from build123d import *

# Parameters (mm, degrees)
F1_DEPTH = 2
F3_DEPTH = 35
F5_DEPTH = 2


with BuildPart() as f1:
    # F0 (on Top) → F1 (new body)
    with BuildSketch(Plane.XY):
        Polygon((-94, 0), (94, 0), (0, 89.7997772826), align=None)
    extrude(amount=F1_DEPTH)

    # F2 (on face) → F3 (join)
    with BuildSketch(Plane.XY.offset(2)):
        Polygon((-91.1046698793, 0), (0, 87.0338198358), (91.1046698793, 0), (94, 0), (0, 89.7997772826), (-94, 0), align=None)
    extrude(amount=F3_DEPTH)

    # F4 (on face) → F5 (join)
    with BuildSketch(Plane.XY.offset(37)):
        Polygon((-91.1046698793, 0), (91.1046698793, 0), (0, 87.0338198358), align=None)
        Polygon((91.1046698793, 0), (94, 0), (0, 89.7997772826), (-94, 0), (-91.1046698793, 0), (0, 87.0338198358), align=None)
    extrude(amount=F5_DEPTH)


solid = f1.part
Build history of the part. All positions in model axes, mm. A direction names the side the tool comes from. Give positions to 0.01 mm unless a question says otherwise; leave off trailing zeros. Order: outer loops, then holes, each group sorted by start corner. A loop starts at its lowest first (then second) coordinate and runs counter-clockwise, first axis right, second up. Notation, with made-up numbers: M 62,-39.5 L 115,-39.5 A14 ccw 115,-35.5 Z; hole C -8.75,-18.75 d5. An arc over 180 degrees is marked long. Put each result on its own line as item: value.
Item 1: Drop flat-ended pins along their axis: pin 1 Ø8 at (y, z) = (10.5, 31.5) entering from -X; pin 2 Ø1 at (y, z) = (73.5, 26) entering from +X; pin 3 Ø6 at (y, z) = (74, 18) entering from -X. Give the stop position or say it passes through.
Results are:
pin 1: x = -87.2
pin 2: x = 17.59
pin 3: x = -19.68
Item 2: Cut at B-B on z = 9. Write the cut outline in (x, y).
Results are:
outline: M -94,0 L -91.1,0 L 0,87.03 L 91.1,0 L 94,0 L 0,89.8 Z
Item 3: Cut at D-D on y = 25. Write the cut outline in (x, z), then the cut area to 3 significant figures.
Results are:
outline: M -67.83,0 L 67.83,0 L 67.83,39 L -67.83,39 Z; hole M -64.94,2 L 64.94,2 L 64.94,37 L -64.94,37 Z
area: 745 mm2
Item 4: Which spindle directions (+Z, -Z, +X, -X, +Y, -Y) get a long thin tool onto all of the face, cutting with end or side? Do faces 5 (the face through (-46.2, 42.9, 19.3)), 6 (the face through (-1, 36, 0)). Say none if no direction does.
Results are:
face 5: -Y
face 6: -Z, +X, -X, +Y, -Y
Item 5: Cut at C-C on x = 35. Write the cut outline in (y, z), then the cut area to 3 significant figures.
Results are:
outline: M 0,0 L 56.36,0 L 56.36,39 L 0,39 L 0,37 L 53.6,37 L 53.6,2 L 0,2 Z
area: 322 mm2
Item 6: Wall check: probe 1 along Z at (x, y) = (38, 33.5); probe 2 along X at (y, z) = (18.5, 33.5); probe 3 along X at (y, z) = (32.5, 36). Give the ranges that are in metal, low to high.
Results are:
probe 1: 0 to 2, 37 to 39
probe 2: -74.63 to -71.74, 71.74 to 74.63
probe 3: -59.98 to -57.08, 57.08 to 59.98
Item 7: Cut at A-A on y = 52. Write the cut outline in (x, z), then the cut area to 3 significant figures.
Results are:
outline: M -39.57,0 L 39.57,0 L 39.57,39 L -39.57,39 Z; hole M -36.67,2 L 36.67,2 L 36.67,37 L -36.67,37 Z
area: 519 mm2
Item 8: Pull direction X, two halves, no side cores. Call faces 1 (the face through (-1, 34, 37)), 2 (the face through (-1, 36, 39)), 3 (the face through (47.66, 44.27, 19.23)), 4 (the face through (-1, 34, 2)): +X half, -X half, draft (parallel to the pull), parting line (faces both ways), or undercut.
Results are:
face 1: undercut
face 2: draft
face 3: +X half
face 4: undercut
